Autodesk Inventor part; units mm, degrees
ref_plane "YZ Plane" through (0, 0, 0) normal (1, 0, 0) x (0, 1, 0)
ref_plane "XZ Plane" through (0, 0, 0) normal (0, 1, 0) x (-1, 0, 0)
ref_plane "XY Plane" through (0, 0, 0) normal (0, 0, 1) x (1, 0, 0)
sketch "Sketch1" plane through (0, 0, 0) normal (0, 0, 1) x (1, 0, 0)
  line L0 (-25.35, 25.35) -> (25.35, 25.35)
  line L1 (25.35, 25.35) -> (25.35, -25.35)
  line L2 (25.35, -25.35) -> (-25.35, -25.35)
  line L3 (-25.35, -25.35) -> (-25.35, 25.35)
  line L4 (-25.35, 25.35) -> (25.35, -25.35) construction
  line L5 (25.35, 25.35) -> (-25.35, -25.35) construction
  line L6 (-41.35, 41.35) -> (41.35, 41.35)
  line L7 (41.35, 41.35) -> (41.35, -41.35)
  line L8 (41.35, -41.35) -> (-41.35, -41.35)
  line L9 (-41.35, -41.35) -> (-41.35, 41.35)
  line L10 (-41.35, 41.35) -> (41.35, -41.35) construction
  line L11 (41.35, 41.35) -> (-41.35, -41.35) construction
  line L12 (-33.35, -33.35) -> (33.35, -33.35) construction
  line L13 (33.35, -33.35) -> (33.35, 33.35) construction
  line L14 (33.35, 33.35) -> (-33.35, 33.35) construction
  line L15 (-33.35, 33.35) -> (-33.35, -33.35) construction
  line L16 (-33.35, -33.35) -> (33.35, 33.35) construction
  line L17 (33.35, -33.35) -> (-33.35, 33.35) construction
  circle A0 centre (-33.35, 33.35) radius 2.9
  circle A1 centre (33.35, 33.35) radius 2.9
  circle A2 centre (33.35, -33.35) radius 2.9
  circle A3 centre (-33.35, -33.35) radius 2.9
  point P0 (0, 0)
  dimension "d0" = 50.7
  dimension "d1" = 50.7
  dimension "d2" = 16
  dimension "d3" = 8
  dimension "d4" = 16
  dimension "d5" = 5.8
extrude "Extrusion1" add sketch "Sketch1" along normal blind 1.7
sketch "Sketch2" plane through (0, 0, 0) normal (0, 0, -1) x (-1, 0, 0)
  line L0 (-25.35, -25.35) -> (-25.35, 25.35)
  line L1 (-25.35, 25.35) -> (25.35, 25.35)
  line L2 (25.35, 25.35) -> (25.35, -25.35)
  line L3 (25.35, -25.35) -> (-25.35, -25.35)
  circle A0 centre (33.35, -33.35) radius 2.9
  circle A1 centre (-33.35, -33.35) radius 2.9
  circle A2 centre (-33.35, 33.35) radius 2.9
  circle A3 centre (33.35, 33.35) radius 2.9
  line L4 (41.35, 41.35) -> (-41.35, 41.35)
  line L5 (-41.35, 41.35) -> (-41.35, -41.35)
  line L6 (-41.35, -41.35) -> (41.35, -41.35)
  line L7 (41.35, -41.35) -> (41.35, 41.35)
  line L8 (-24.55, 21.35) -> (-24.55, 2.35)
  line L9 (-17.35, -23.35) -> (17.35, -23.35)
  line L10 (19.35, -21.35) -> (19.35, -2)
  line L11 (23.35, 23.35) -> (-22.55, 23.35)
  line L12 (21.35, 0) -> (23.35, 0)
  line L13 (-22.55, 0.35) -> (-21.35, 0.35)
  line L14 (-19.35, -1.65) -> (-19.35, -21.35)
  arc A4 (-22.55, 23.35) -> (-24.55, 21.35) centre (-22.55, 21.35) ccw
  arc A5 (-24.55, 2.35) -> (-22.55, 0.35) centre (-22.55, 2.35) ccw
  arc A6 (-19.35, -1.65) -> (-21.35, 0.35) centre (-21.35, -1.65) ccw
  arc A7 (-19.35, -21.35) -> (-17.35, -23.35) centre (-17.35, -21.35) ccw
  arc A8 (17.35, -23.35) -> (19.35, -21.35) centre (17.35, -21.35) ccw
  arc A9 (21.35, 0) -> (19.35, -2) centre (21.35, -2) ccw
  line L15 (25.35, 21.35) -> (25.35, 2)
  arc A10 (25.35, 21.35) -> (23.35, 23.35) centre (23.35, 21.35) ccw
  arc A11 (23.35, 0) -> (25.35, 2) centre (23.35, 2) ccw
  point P0 (0, 0)
  point P1 (25.35, 23.35)
  point P2 (25.35, 0)
  dimension "d8" = 0.8
  dimension "d9" = 6
  dimension "d10" = 6
  dimension "d11" = 2
  dimension "d12" = 2
  dimension "d13" = 41
  dimension "d14" = 2
  dimension "d15" = 2
extrude "Extrusion2" add sketch "Sketch2" along normal blind 1.7 contours L0 L1 L2 A10 L11 A4 L8 A5 L13 A6 L14 A7 L9 A8 L10 A9 L12 A11 L3 | L7 L6 L5 L4
fillet "Fillet1" radius 1 12 edges at (0, 41.35, 1.7) (-41.35, 0, 1.7) (0, -41.35, 1.7) (41.35, 0, 1.7) (0, 41.35, -1.7) (41.35, 0, -1.7) (0, -41.35, -1.7) (-41.35, 0, -1.7) (25.35, 0, 1.7) (0, -25.35, 1.7) (-25.35, 0, 1.7) (0, 25.35, 1.7)
fillet "Fillet2" radius 1 12 edges at (-41.0571, -41.0571, -1.4071) (-41.0571, -41.0571, 1.4071) (-41.35, -41.35, 0) (41.35, -41.35, 0) (41.0571, -41.0571, -1.4071) (41.0571, -41.0571, 1.4071) (41.35, 41.35, 0) (41.0571, 41.0571, -1.4071) (41.0571, 41.0571, 1.4071) (-41.0571, 41.0571, 1.4071) (-41.0571, 41.0571, -1.4071) (-41.35, 41.35, 0)
equation "\"d3\" = 0.5 * d2"
equation "\"d4\" = d2"
equation "\"d10\" = d9"
equation "\"d11\" = d12"
properties part number "Jig_Power"
Geometry: final body of the model. Coordinates: model frame, mm. A direction names the side the tool comes from. Coordinates: 2 decimals unless noted, no trailing zeros. Order: outer loops, then holes, each group sorted by start corner. A loop starts at its lowest first (then second) coordinate and runs counter-clockwise, first axis right, second up.
1) Section A-A (x = 33.35). Return loops of the section in (y, z).
Result sheet:
outline: (-41.35, -0.7) arc R1 ccw to (-40.35, -1.7) - (-36.25, -1.7) - (-36.25, 1.7) - (-40.35, 1.7) arc R1 ccw to (-41.35, 0.7) - close; (-30.45, -1.7) - (30.45, -1.7) - (30.45, 1.7) - (-30.45, 1.7) - close; (36.25, -1.7) - (40.35, -1.7) arc R1 ccw to (41.35, -0.7) - (41.35, 0.7) arc R1 ccw to (40.35, 1.7) - (36.25, 1.7) - close
2) Section C-C (y = 4). Return loops of the section in (x, z).
Result sheet:
outline: (-41.35, -0.7) arc R1 ccw to (-40.35, -1.7) - (-25.35, -1.7) - (-25.35, 0.7) arc R1 ccw to (-26.35, 1.7) - (-40.35, 1.7) arc R1 ccw to (-41.35, 0.7) - close; (24.55, -1.7) - (40.35, -1.7) arc R1 ccw to (41.35, -0.7) - (41.35, 0.7) arc R1 ccw to (40.35, 1.7) - (26.35, 1.7) arc R1 ccw to (25.35, 0.7) - (25.35, 0) - (24.55, 0) - close
3) Section D-D (x = -5). Return loops of the section in (y, z), then the cut area to 3 significant figures.
Result sheet:
outline: (-41.35, -0.7) arc R1 ccw to (-40.35, -1.7) - (-23.35, -1.7) - (-23.35, 0) - (-25.35, 0) - (-25.35, 0.7) arc R1 ccw to (-26.35, 1.7) - (-40.35, 1.7) arc R1 ccw to (-41.35, 0.7) - close; (23.35, -1.7) - (40.35, -1.7) arc R1 ccw to (41.35, -0.7) - (41.35, 0.7) arc R1 ccw to (40.35, 1.7) - (26.35, 1.7) arc R1 ccw to (25.35, 0.7) - (25.35, 0) - (23.35, 0) - close
area: 114 mm2
4) Set-up query: faces 1 (the flat face through (0, -24, 0)), 2 (the flat face through (27, 1, -1.7)), 3 (the cylindrical face through (-24.75, 22.78, -0.84)). Return all of +Z, -Z, +X, -X, +Y, -Y with unobstructed straight access to the full face (end or side cutting, diameter ignored); none if empty.
Result sheet:
face 1: +Z
face 2: -Z, +X, -X, +Y, -Y
face 3: +Z, -Z
5) Draft query along Y for faces 4 (the flat face through (-10, 27, 1.7)), 5 (the cylindrical face through (23.98, 22.75, -0.84)). Return one class per face: released by +Y, released by -Y, zero draft, split by the parting line, or undercut.
Result sheet:
face 4: zero draft
face 5: undercut
6) Ray query, probe 1 along X at (y, z) = (33.35, -0.6); probe 2 along X at (y, z) = (-33.35, 0.9); probe 3 along Y at (x, z) = (-33.35, 0.8). Return the intervals inside material, ascending.
Result sheet:
probe 1: x = -41.35 to -36.25, -30.45 to 30.45, 36.25 to 41.35
probe 2: x = -41.33 to -36.25, -30.45 to 30.45, 36.25 to 41.33
probe 3: y = -41.34 to -36.25, -30.45 to 30.45, 36.25 to 41.34
7) First-contact query: P1, Ø0.5, axis at y = -13.5, z = -1.5, coming from the +X side; P2, Ø4.5, axis at x = -33.35, y = -33.35, coming from the +Z side; P3, Ø6, axis at x = 16.5, y = -18.5, coming from the +Z side. Flat tips, straight axial feed; report the tip coordinate or a pass-through.
Result sheet:
P1: stops at x = 41.19
P2: passes through
P3: stops at z = 0
